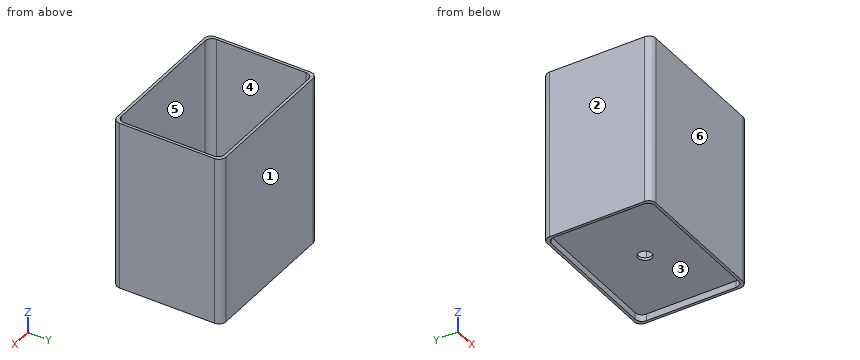
from build123d import *

# Parameters (mm, degrees)
F1_DEPTH = 152.4
F2_DEPTH = 6.35
F3_DEPTH = 2.54
F4_D     = 12.7


with BuildPart() as f1:
    # F0 (on Top) → F1 (new body)
    with BuildSketch(Plane.XY):
        with BuildLine():
            Line((63.5, 50.8), (-63.5, 50.8))
            ThreePointArc((-63.5, 50.8), (-67.990128, 48.940128), (-69.85, 44.45))
            Line((-69.85, 44.45), (-69.85, -44.45))
            ThreePointArc((-69.85, -44.45), (-67.990128, -48.940128), (-63.5, -50.8))
            Line((-63.5, -50.8), (63.5, -50.8))
            ThreePointArc((63.5, -50.8), (67.990128, -48.940128), (69.85, -44.45))
            Line((69.85, -44.45), (69.85, 44.45))
            ThreePointArc((69.85, 44.45), (67.990128, 48.940128), (63.5, 50.8))
        make_face()
        with BuildLine():
            ThreePointArc((-67.31, 41.91), (-65.450128, 46.400128), (-60.96, 48.26))
            Line((-60.96, 48.26), (60.96, 48.26))
            ThreePointArc((60.96, 48.26), (65.450128, 46.400128), (67.31, 41.91))
            Line((67.31, 41.91), (67.31, -41.91))
            ThreePointArc((67.31, -41.91), (65.450128, -46.400128), (60.96, -48.26))
            Line((60.96, -48.26), (-60.96, -48.26))
            ThreePointArc((-60.96, -48.26), (-65.450128, -46.400128), (-67.31, -41.91))
            Line((-67.31, -41.91), (-67.31, 41.91))
        make_face(mode=Mode.SUBTRACT)
    extrude(amount=F1_DEPTH)

    # F0 (on Top) → F2 (join)
    with BuildSketch(Plane.XY):
        with BuildLine():
            Line((63.5, 50.8), (-63.5, 50.8))
            ThreePointArc((-63.5, 50.8), (-67.990128, 48.940128), (-69.85, 44.45))
            Line((-69.85, 44.45), (-69.85, -44.45))
            ThreePointArc((-69.85, -44.45), (-67.990128, -48.940128), (-63.5, -50.8))
            Line((-63.5, -50.8), (63.5, -50.8))
            ThreePointArc((63.5, -50.8), (67.990128, -48.940128), (69.85, -44.45))
            Line((69.85, -44.45), (69.85, 44.45))
            ThreePointArc((69.85, 44.45), (67.990128, 48.940128), (63.5, 50.8))
        make_face()
        with BuildLine():
            ThreePointArc((-67.31, 41.91), (-65.450128, 46.400128), (-60.96, 48.26))
            Line((-60.96, 48.26), (60.96, 48.26))
            ThreePointArc((60.96, 48.26), (65.450128, 46.400128), (67.31, 41.91))
            Line((67.31, 41.91), (67.31, -41.91))
            ThreePointArc((67.31, -41.91), (65.450128, -46.400128), (60.96, -48.26))
            Line((60.96, -48.26), (-60.96, -48.26))
            ThreePointArc((-60.96, -48.26), (-65.450128, -46.400128), (-67.31, -41.91))
            Line((-67.31, -41.91), (-67.31, 41.91))
        make_face(mode=Mode.SUBTRACT)
    extrude(amount=-F2_DEPTH)

    # F0 (on Top) → F3 (join)
    with BuildSketch(Plane.XY):
        with BuildLine():
            Line((60.96, 48.26), (-60.96, 48.26))
            ThreePointArc((-60.96, 48.26), (-65.450128, 46.400128), (-67.31, 41.91))
            Line((-67.31, 41.91), (-67.31, -41.91))
            ThreePointArc((-67.31, -41.91), (-65.450128, -46.400128), (-60.96, -48.26))
            Line((-60.96, -48.26), (60.96, -48.26))
            ThreePointArc((60.96, -48.26), (65.450128, -46.400128), (67.31, -41.91))
            Line((67.31, -41.91), (67.31, 41.91))
            ThreePointArc((67.31, 41.91), (65.450128, 46.400128), (60.96, 48.26))
        make_face()
    extrude(amount=F3_DEPTH)

    # F4 (through all)
    with Locations(Plane(origin=(0, 0, 0), x_dir=(1, 0, 0), z_dir=(0, 0, -1))):
        with Locations((0, 0)):
            Hole(F4_D / 2)


solid = f1.part
The listing builds one solid part. Answer for the finished solid, in the listing's coordinates (mm). Face numbers are marked on the shaded views. A direction names the side the tool comes from. Give positions to 0.01 mm unless a question says otherwise; leave off trailing zeros. Loops run counter-clockwise (first coordinate to the right, second up) from the corner with the lowest first, then second, coordinate; pieces in that order, holes last.
Item 1: Find the intervals of material crossed by line 1 along Y through (x, z) = (0, 0.8); line 2 along Y through (x, z) = (51, 51); line 3 along X through (y, z) = (31, 83.5), in increasing order.
Derived:
line 1: y = -50.8 to -6.35, 6.35 to 50.8
line 2: y = -50.8 to -48.26, 48.26 to 50.8
line 3: x = -69.85 to -67.31, 67.31 to 69.85
Item 2: Determine the mould class of the marked faces 1, 2, 3 and 4 for opening direction Y: +Y half, -Y half, draft (parallel to the pull), parting line (faces both ways), or undercut.
Derived:
face 1: +Y half
face 2: draft
face 3: undercut
face 4: undercut
Item 3: A cutting plane is placed at D-D (x = 37.5). Give the vertices of the cut face in (y, z), then the cut area to 3 significant figures.
Derived:
outline: (-50.8, -6.35) - (-48.26, -6.35) - (-48.26, 0) - (48.26, 0) - (48.26, -6.35) - (50.8, -6.35) - (50.8, 152.4) - (48.26, 152.4) - (48.26, 2.54) - (-48.26, 2.54) - (-48.26, 152.4) - (-50.8, 152.4) - close
area: 1,050 mm2
Item 4: A cutting plane is placed at B-B (z = 108.5). Give the vertices of the cut face in (x, y), then the cut area to 3 significant figures.
Derived:
outline: (-69.85, -44.45) arc R6.35 ccw to (-63.5, -50.8) - (63.5, -50.8) arc R6.35 ccw to (69.85, -44.45) - (69.85, 44.45) arc R6.35 ccw to (63.5, 50.8) - (-63.5, 50.8) arc R6.35 ccw to (-69.85, 44.45) - close; hole (-67.31, -41.91) arc R6.35 ccw to (-60.96, -48.26) - (60.96, -48.26) arc R6.35 ccw to (67.31, -41.91) - (67.31, 41.91) arc R6.35 ccw to (60.96, 48.26) - (-60.96, 48.26) arc R6.35 ccw to (-67.31, 41.91) - close
area: 1,200 mm2
Item 5: A cutting plane is placed at A-A (y = 0). Give the vertices of the cut face in (x, z).
Derived:
outline: (-69.85, -6.35) - (-67.31, -6.35) - (-67.31, 0) - (-6.35, 0) - (-6.35, 2.54) - (-67.31, 2.54) - (-67.31, 152.4) - (-69.85, 152.4) - close; (6.35, 0) - (67.31, 0) - (67.31, -6.35) - (69.85, -6.35) - (69.85, 152.4) - (67.31, 152.4) - (67.31, 2.54) - (6.35, 2.54) - close
Item 6: A tool of negligible diameter and unlimited length cuts with its end or side. For the marked faces 5 and 6, from which of +Z, -Z, +X, -X, +Y, -Y can it reach the whole face along a straight path? Write none if from no direction.
Derived:
face 5: +Z
face 6: +Z, -Z, +X, -X, -Y
Item 7: A cutting plane is placed at C-C (x = 0). Give the vertices of the cut face in (y, z), then the cut area to 3 significant figures.
Derived:
outline: (-50.8, -6.35) - (-48.26, -6.35) - (-48.26, 0) - (-6.35, 0) - (-6.35, 2.54) - (-48.26, 2.54) - (-48.26, 152.4) - (-50.8, 152.4) - close; (6.35, 0) - (48.26, 0) - (48.26, -6.35) - (50.8, -6.35) - (50.8, 152.4) - (48.26, 152.4) - (48.26, 2.54) - (6.35, 2.54) - close
area: 1,020 mm2
Item 8: This flat-tipped pin is pushed along its axis until it touches: pin 1 Ø10 at (x, y) = (-30, -31) entering from -Z. Where does it stop, or does it pass through?
Derived:
pin 1: stops at z = 0
